Part print with two shaded views. Sizes in mm from the minimum x, y, z corner. A direction names the side the tool comes from. Round coordinates to 2 decimals unless told otherwise and drop trailing zeros. Write each loop counter-clockwise with the first axis right and the second up, starting at its lowest first coordinate (ties: lowest second). Pieces come first, ordered by that corner, then holes.
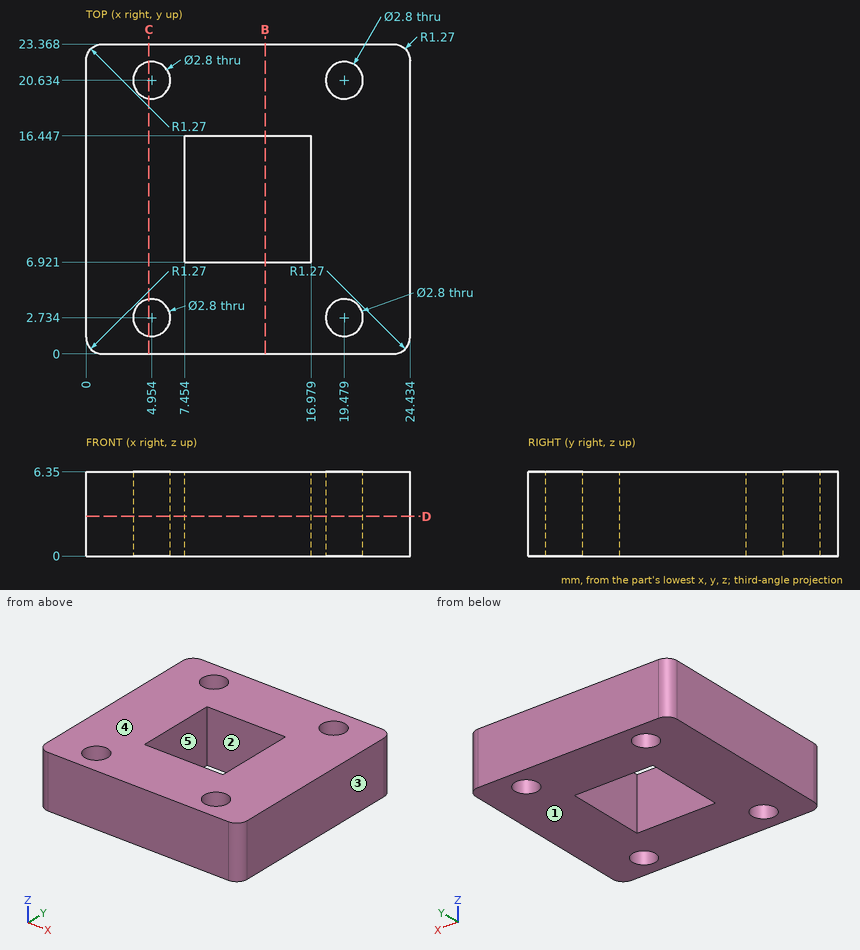
Q1. Cut at C-C on x = 4.75. Write the cut outline in (y, z).
Values follow:
outline: (0, 0) - (1.35, 0) - (1.35, 6.35) - (0, 6.35) - close; (4.12, 0) - (19.25, 0) - (19.25, 6.35) - (4.12, 6.35) - close; (22.02, 0) - (23.37, 0) - (23.37, 6.35) - (22.02, 6.35) - close
Q2. Drop a flat-ended pin along its axis: pin 1 (1.7 mm diameter, centred on x = 19.48, y = 20.63, fed in from -Z). Give the stop position or say it passes through.
Values follow:
pin 1: passes through
Q3. Wall check: L1, parallel to Y at x = 5, z = 1.25 (1 decimal); L2, parallel to X at y = 15.75, z = 3 (1 decimal); L3, parallel to Y at x = 14.5, z = 5. Give the ranges that are in metal, low to high.
Values follow:
L1: y = 0 to 1.3, 4.1 to 19.2, 22 to 23.4
L2: x = 0 to 7.5, 17 to 24.4
L3: y = 0 to 6.92, 16.45 to 23.37
Q4. Mould opens along X. For the marked faces 1, 2 and 3 say: +X half, -X half, draft (parallel to the pull), parting line (faces both ways), or undercut.
Values follow:
face 1: draft
face 2: undercut
face 3: +X half
Q5. Which spindle directions (+Z, -Z, +X, -X, +Y, -Y) get a long thin tool onto all of the face, cutting with end or side? Do the marked faces 4 and 5. Say none if no direction does.
Values follow:
face 4: +Z, +X, -X, +Y, -Y
face 5: +Z, -Z
Q6. Cut at B-B on x = 13.5. Write the cut outline in (y, z).
Values follow:
outline: (0, 0) - (6.92, 0) - (6.92, 6.35) - (0, 6.35) - close; (16.45, 0) - (23.37, 0) - (23.37, 6.35) - (16.45, 6.35) - close
Q7. Cut at D-D on z = 3. Write the cut outline in (x, y) (1 decimal), plus the area to 3 significant figures.
Values follow:
outline: (0, 1.3) arc R1.3 ccw to (1.3, 0) - (23.2, 0) arc R1.3 ccw to (24.4, 1.3) - (24.4, 22.1) arc R1.3 ccw to (23.2, 23.4) - (1.3, 23.4) arc R1.3 ccw to (0, 22.1) - close; hole circle Ø2.8 at (5, 2.7); hole circle Ø2.8 at (5, 20.6); hole (7.5, 6.9) - (17, 6.9) - (17, 16.4) - (7.5, 16.4) - close; hole circle Ø2.8 at (19.5, 2.7); hole circle Ø2.8 at (19.5, 20.6)
area: 454 mm2
